Geometry check sheet. Reference: the model listing, model coordinates, mm. A direction names the side the tool comes from. Round coordinates to 2 decimals unless told otherwise and drop trailing zeros. Write each loop counter-clockwise with the first axis right and the second up, starting at its lowest first coordinate (ties: lowest second). Pieces come first, ordered by that corner, then holes. Notation, with made-up numbers: (14, 62.5) -> (67, 62.5) arc R4 cw to (67, 68.5) -> close; hole circle Ø7 at (-15, -38). An arc over 180 degrees is marked (long way). Use a Markdown table: item, result.
```python
from build123d import *

# Parameters (mm, degrees)
SKETCH1_R                   = 15.748
BOSS_EXTRUDE1_DEPTH         = 12.7
F_1_1_DIAMETER_HOLE1_D      = 25.4
F_1_1_DIAMETER_HOLE1_DEPTH  = 10.16
F_1_1_DIAMETER_HOLE1_TIP    = 7.630929862
F_3_4_0_75_DIAMETER_HOLE1_D = 19.05


with BuildPart() as part:
    # Sketch1 → Boss-Extrude1 (new body)
    with BuildSketch(Plane(origin=(0, 0, 0), x_dir=(1, 0, 0), z_dir=(0, 1, 0))):
        Circle(SKETCH1_R)
    extrude(amount=BOSS_EXTRUDE1_DEPTH)

    # 1 (1) Diameter Hole1
    with Locations(Plane.ZX.offset(12.7)):
        with Locations((0, 0)):
            Hole(F_1_1_DIAMETER_HOLE1_D / 2, depth=F_1_1_DIAMETER_HOLE1_DEPTH)
            with Locations((0, 0, -(F_1_1_DIAMETER_HOLE1_DEPTH + F_1_1_DIAMETER_HOLE1_TIP / 2))):  # 118° drill point
                Cone(0, F_1_1_DIAMETER_HOLE1_D / 2, F_1_1_DIAMETER_HOLE1_TIP, mode=Mode.SUBTRACT)

    # 3/4 (0.75) Diameter Hole1 (through all)
    with Locations(Plane.ZX.offset(12.7)):
        with Locations((0, 0)):
            Hole(F_3_4_0_75_DIAMETER_HOLE1_D / 2)


solid = part.part
```
(1) Section check B-B on x = 0. Record the cut outline in (y, z) (3 decimals), plus the area to 3 significant figures.
A:
| item | result |
|---|---|
| outline | (0, -15.748) -> (12.7, -15.748) -> (12.7, -12.7) -> (2.54, -12.7) -> (0.632, -9.525) -> (0, -9.525) -> close; (0, 9.525) -> (0.632, 9.525) -> (2.54, 12.7) -> (12.7, 12.7) -> (12.7, 15.748) -> (0, 15.748) -> close |
| area | 87.5 mm2 |
(2) Access from +Z, -Z, +X, -X, +Y, -Y to the whole of each face (thin tool, end or side, straight path). Record for faces 5 (the face through (-11, 12.7, -7)), 6 (the face through (-12.4, 7.55, 2.75)).
A:
| item | result |
|---|---|
| face 5 | +Z, -Z, +X, -X, +Y |
| face 6 | +Y |
(3) Gauge pin test, flat ends, axial feed: pin 1 Ø10 at (x, z) = (7.5, 1) entering from +Y; pin 2 Ø11.5 at (x, z) = (0, 0) entering from -Y; pin 3 Ø2 at (x, y) = (2.5, 4.5) entering from +Z; pin 4 Ø2 at (y, z) = (11.5, 3.5) entering from -X. Record the tip position at first contact, or that the pin passes through.
A:
| item | result |
|---|---|
| pin 1 | stops at y = 2.46 |
| pin 2 | passes through |
| pin 3 | stops at z = 15.68 |
| pin 4 | stops at x = -15.55 |
(4) Section check A-A on z = 0. Record the cut outline in (x, y) (3 decimals), plus the area to 3 significant figures.
A:
| item | result |
|---|---|
| outline | (-15.748, 0) -> (-9.525, 0) -> (-9.525, 0.632) -> (-12.7, 2.54) -> (-12.7, 12.7) -> (-15.748, 12.7) -> close; (9.525, 0) -> (15.748, 0) -> (15.748, 12.7) -> (12.7, 12.7) -> (12.7, 2.54) -> (9.525, 0.632) -> close |
| area | 87.5 mm2 |
(5) Release check for a two-part mould opening along Z. For faces 1 (the face through (-9.49, 0.75, -2.11)), 2 (the face through (-3.414, 6.261, 15.374)), 3 (the face through (7, 0, 7)), 4 (the face through (-5.796, 0.312, 7.559)) record: +Z half, -Z half, draft (parallel to the pull), parting line (faces both ways), or undercut.
A:
| item | result |
|---|---|
| face 1 | undercut |
| face 2 | parting line |
| face 3 | draft |
| face 4 | undercut |
(6) Section check C-C on y = 3. Record the cut outline in (x, z), plus the area to 3 significant figures.
A:
| item | result |
|---|---|
| outline | circle Ø31.5 at (0, 0); hole circle Ø25.4 at (0, 0) |
| area | 272 mm2 |
(7) Thickness scan on line 1 (X direction, y = 0.2, z = 0) (3 decimals); line 2 (Z direction, x = 0, y = 7.25). Record the ranges inside material, lowest first.
A:
| item | result |
|---|---|
| line 1 | x = -15.748 to -9.525, 9.525 to 15.748 |
| line 2 | z = -15.75 to -12.7, 12.7 to 15.75 |
(8) Section check D-D on x = 13.5. Record the cut outline in (y, z), plus the area to 3 significant figures.
A:
| item | result |
|---|---|
| outline | (0, -8.11) -> (12.7, -8.11) -> (12.7, 8.11) -> (0, 8.11) -> close |
| area | 206 mm2 |
